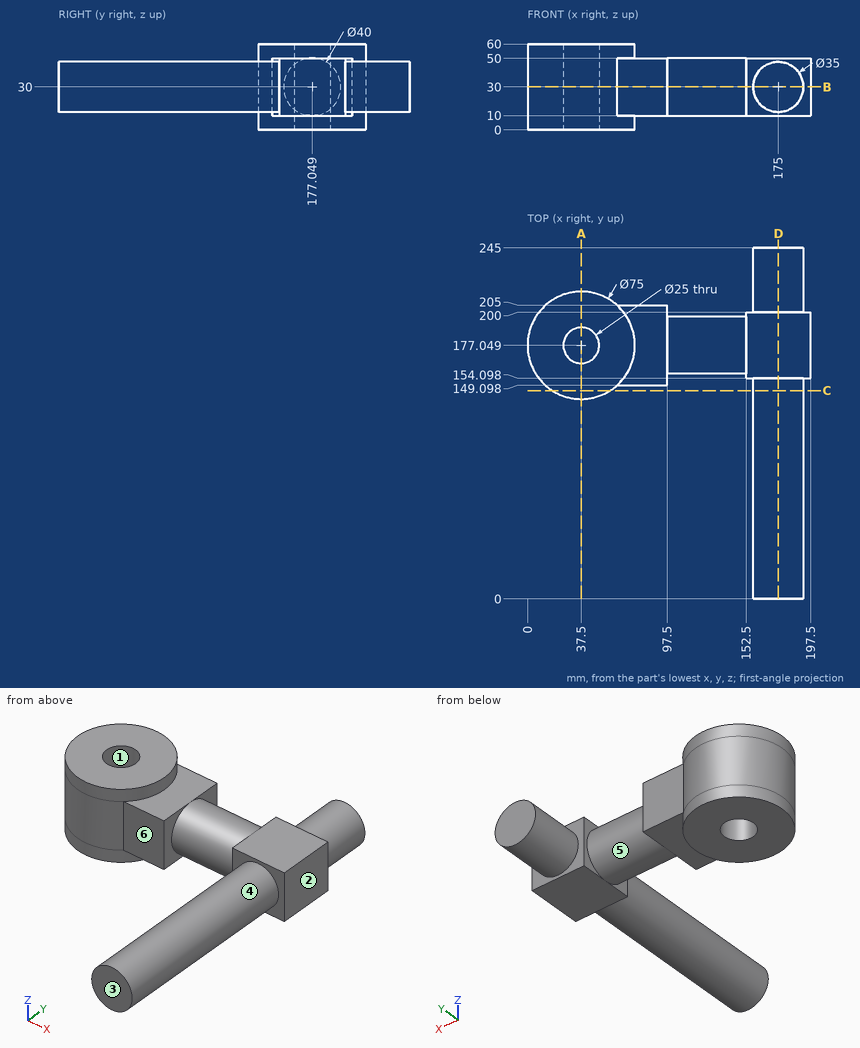
Can you work these out from the drawing? Everything is in mm from the part's minimum corner. A direction names the side the tool comes from. Coordinates: 2 decimals unless noted, no trailing zeros. Loops run counter-clockwise (first coordinate to the right, second up) from the corner with the lowest first, then second, coordinate; pieces in that order, holes last. Notation, with made-up numbers: (-38.75, 30.25) - (-27.75, 30.25) arc R25 ccw to (-27.75, 69.25) - close; hole circle Ø1 at (12, 70). An arc over 180 degrees is marked (long way). Put each result on its own line as item: value. Start each with the question number.
Item 1: If we mould it in two halves opening along X, with no side actions, what happens to the marked faces 1, 2 and 3? For each: +X half, -X half, draft (parallel to the pull), parting line (faces both ways), or undercut.
Item 2: Suppose I cut it at A-A (x = 37.5). Please give me the cut outline in (y, z), and give its area (3 significant figures).
Item 3: If I drill on line 1 along Y through (x, z) = (37.5, 47); line 2 along X through (y, z) = (102.5, 30.5); line 3 along X through (y, z) = (184.5, 6), over which ranges is the centre line in solid material (lowest first)?
Item 4: Suppose I cut it at D-D (x = 175). Please give me the cut outline in (y, z), and give its area (3 significant figures).
Item 5: Suppose I cut it at C-C (y = 145.5). Please give me the cut outline in (x, z).
Item 6: Suppose I cut it at B-B (z = 30). Please give me the cut outline in (x, y), and give its area (3 significant figures).
Item 7: Which directions (+Z, -Z, +X, -X, +Y, -Y) give clear straight access to the entire face, cutting with the end or side of a thin tool? Please do the marked faces 4, 5 and 6.
Item 8: For pin 1 (10.5 mm diameter, centred on x = 75, z = 27.5, fed in from +Y); pin 2 (17.5 mm diameter, centred on x = 77, z = 20.5, fed in from -Y); pin 3 (7 mm diameter, centred on y = 183.5, z = 25.5, fed in from -X), each with a flat end and sliding along its axis, tell me the tip position at first contact or that it passes through.
Here are the results:
1. face 1: undercut
1. face 2: +X half
1. face 3: draft
2. outline: (139.55, 0) - (164.55, 0) - (164.55, 60) - (139.55, 60) - close; (189.55, 0) - (214.55, 0) - (214.55, 60) - (189.55, 60) - close
2. area: 3,000 mm²
3. line 1: 139.55 to 164.55, 189.55 to 214.55
3. line 2: 157.51 to 192.49
3. line 3: 0.75 to 27.46, 47.54 to 74.25
4. outline: (0, 12.5) - (154.1, 12.5) - (154.1, 10) - (200, 10) - (200, 12.5) - (245, 12.5) - (245, 47.5) - (200, 47.5) - (200, 50) - (154.1, 50) - (154.1, 47.5) - (0, 47.5) - close
4. area: 8,800 mm²
5. outline: (17.23, 0) - (57.77, 0) - (57.77, 60) - (17.23, 60) - close; circle Ø35 at (175, 30)
6. outline: (62.5, 149.1) - (97.5, 149.1) - (97.5, 157.05) - (152.5, 157.05) - (152.5, 154.1) - (157.5, 154.1) - (157.5, 0) - (192.5, 0) - (192.5, 154.1) - (197.5, 154.1) - (197.5, 200) - (192.5, 200) - (192.5, 245) - (157.5, 245) - (157.5, 200) - (152.5, 200) - (152.5, 197.05) - (97.5, 197.05) - (97.5, 205) - (62.5, 205) arc R37.5 ccw (long way) to start; hole circle Ø25 at (37.5, 177.05)
6. area: 16,600 mm²
7. face 4: -Y
7. face 5: none
7. face 6: +Z, -Z, -Y
8. pin 1: y = 205
8. pin 2: y = 149.1
8. pin 3: x = 0.12
